```python
from build123d import *

# Parameters (mm, degrees)
CROQUIS_BASE_W         = 20.5
CROQUIS_BASE_H         = 21
BRIDA_BASE1_DEPTH      = 2
BRIDA_DE_ARISTA1_DEPTH = 21
CROQUIS11_R            = 3
CROQUIS11_R_2          = 1.5
CORTAR_EXTRUIR1_DEPTH  = 10
CROQUIS12_R            = 1.25
CORTAR_EXTRUIR2_DEPTH  = 2
REDONDEO1_R            = 5


# Sheet-metal steps are written as plain solids
with BuildPart() as part:
    # Croquis base → Brida base1 (new body)
    with BuildSketch(Plane(origin=(0, 0, 0), x_dir=(0, -1, 0), z_dir=(1, 0, 0))):
        Rectangle(CROQUIS_BASE_W, CROQUIS_BASE_H)
    extrude(amount=-BRIDA_BASE1_DEPTH)

    # Brida de arista1 section (across the edge) → Brida de arista1 (add)
    with BuildSketch(Plane(origin=(0, -10.75, 10.5), x_dir=(0, 1, 0), z_dir=(0, 0, -1))):
        with BuildLine():
            Line((-2, 0.5), (-2, 13))
            Line((-2, 13), (0, 13))
            Line((0, 13), (0, 0.5))
            ThreePointArc((0, 0.5), (0.146446609, 0.146446609), (0.5, 0))
            Line((0.5, 0), (0.5, -2))
            ThreePointArc((0.5, -2), (-1.267766953, -1.267766953), (-2, 0.5))
        make_face()
    extrude(amount=BRIDA_DE_ARISTA1_DEPTH)

    # Croquis11 → Cortar-Extruir1 (cut)
    with BuildSketch(Plane(origin=(-2, 0, 0), x_dir=(0, -1, 0), z_dir=(-1, 0, 0))):
        with Locations((0.25, 0)):
            Circle(CROQUIS11_R)
        with Locations((-4.947234842, 5.197234842)):
            Circle(CROQUIS11_R_2)
        with Locations((5.447234842, 5.197234842)):
            Circle(CROQUIS11_R_2)
        with Locations((5.447234842, -5.197234842)):
            Circle(CROQUIS11_R_2)
        with Locations((-4.947234842, -5.197234842)):
            Circle(CROQUIS11_R_2)
    extrude(amount=-CORTAR_EXTRUIR1_DEPTH, mode=Mode.SUBTRACT)

    # Croquis12 → Cortar-Extruir2 (cut)
    with BuildSketch(Plane(origin=(0, -12.75, 0), x_dir=(0, 0, -1), z_dir=(0, -1, 0))):
        with Locations(Location((6, 8, 0), (0, 0, 90))):
            Circle(CROQUIS12_R)
        with Locations(Location((-6, 8, 0), (0, 0, 270))):
            Circle(CROQUIS12_R)
    extrude(amount=-CORTAR_EXTRUIR2_DEPTH, mode=Mode.SUBTRACT)

    # Redondeo1
    redondeo1_edges = [part.edges().sort_by_distance(p)[0] for p in [
        (13, -11.75, 10.5),
        (13, -11.75, -10.5),
        (-1, 10.25, 10.5),
        (-1, 10.25, -10.5),
    ]]
    fillet(redondeo1_edges, radius=REDONDEO1_R)


solid = part.part
```
Input: part model. Units: mm. Frame: model coordinates. A direction names the side the tool comes from. Coordinates: 2 decimals unless noted, no trailing zeros. Write each loop counter-clockwise with the first axis right and the second up, starting at its lowest first coordinate (ties: lowest second). Pieces come first, ordered by that corner, then holes. Notation, with made-up numbers: (-22.5, -6.75) - (10.5, -6.75) arc R22 cw to (10.5, 19.25) - close; hole circle Ø7 at (46, 21). An arc over 180 degrees is marked (long way). Put each result on its own line as item: value. Start each with the question number.
1) Cut plane C-C (z = -6). Return the cut outline in (x, y), plus the area to 3 significant figures.
2) Cut plane B-B (y = -0.25). Return the cut outline in (x, z).
3) Cut plane D-D (y = -4.5). Return the cut outline in (x, z), plus the area to 3 significant figures.
4) Reachability of faces 4 (the face through (11.5, -11.74, 9.07)), 5 (the face through (0, 2.4, -2.5)) from +Z, -Z, +X, -X, +Y, -Y: full face, straight path, thin tool, end or side. Return the list, or none.
5) Contact query for flat-ended pins moving along their axis: pin 1 (5 mm diameter, centred on y = -5.45, z = -5.2, fed in from +X); pin 2 (2.5 mm diameter, centred on y = 4.95, z = -5.2, fed in from +X); pin 3 (4 mm diameter, centred on x = 8, z = -6, fed in from +Y). Output: stop coordinate, or through.
6) Mould query, pull axis Y, two halves, no side actions, for faces 1 (the face through (-1.01, 8.75, 9.07)), 2 (the face through (-1.01, 6.05, -4.18)), 3 (the face through (7, -12.75, 0)). Classes: pulls with the +Y half, pulls with the -Y half, needs draft (parallel to the pull), parting line crosses it, or undercut.
7) Ray query, L1, parallel to Y at x = 3.5, z = 2.75; L2, parallel to X at y = -8.75, z = 4.5; L3, parallel to X at y = -10.5, z = 8.5. Return the intervals inside material, ascending.
8) Cut plane A-A (z = 0). Return the cut outline in (x, y).
Resolved:
1. outline: (-2, -10.25) arc R2.5 ccw to (0.5, -12.75) - (6.75, -12.75) - (6.75, -10.75) - (0.5, -10.75) arc R0.5 cw to (0, -10.25) - (0, -6.71) - (-2, -6.71) - close; (-2, -4.18) - (0, -4.18) - (0, 3.68) - (-2, 3.68) - close; (-2, 6.21) - (0, 6.21) - (0, 10.22) - (-2, 10.22) - close; (9.25, -12.75) - (12.97, -12.75) - (12.97, -10.75) - (9.25, -10.75) - close
1. area: 55.5 mm2
2. outline: (-2, -10.5) - (0, -10.5) - (0, -3) - (-2, -3) - close; (-2, 3) - (0, 3) - (0, 10.5) - (-2, 10.5) - close
3. outline: (-2, -10.5) - (0, -10.5) - (0, -6.36) - (-2, -6.36) - close; (-2, -4.03) - (0, -4.03) - (0, 4.03) - (-2, 4.03) - close; (-2, 6.36) - (0, 6.36) - (0, 10.5) - (-2, 10.5) - close
3. area: 32.7 mm2
4. face 4: +Z, +X, +Y, -Y
4. face 5: +Z, -Z, +X, +Y
5. pin 1: stops at x = 0
5. pin 2: passes through
5. pin 3: stops at y = -10.75
6. face 1: pulls with the +Y half
6. face 2: undercut
6. face 3: pulls with the -Y half
7. L1: y = -12.75 to -10.75
7. L2: x = -2 to 0
7. L3: x = -1.99 to 0.07
8. outline: (-2, -10.25) arc R2.5 ccw to (0.5, -12.75) - (13, -12.75) - (13, -10.75) - (0.5, -10.75) arc R0.5 cw to (0, -10.25) - (0, -3.25) - (-2, -3.25) - close; (-2, 2.75) - (0, 2.75) - (0, 10.25) - (-2, 10.25) - close
